Read the model definition and answer for the solid it produces. Units are mm, in the model's axes. A direction names the side the tool comes from. Round coordinates to 2 decimals unless told otherwise and drop trailing zeros. Write each loop counter-clockwise with the first axis right and the second up, starting at its lowest first coordinate (ties: lowest second). Pieces come first, ordered by that corner, then holes. Notation, with made-up numbers: (61.5, -22.75) -> (84.5, -22.75) arc R21 cw to (84.5, -9.75) -> close; hole circle Ø7 at (24.25, -25.75). An arc over 180 degrees is marked (long way). Return JSON: item names as keys, results as strings.
from build123d import *

# Parameters (mm, degrees)
F1_DEPTH = 8
F2_W     = 110
F2_H     = 20
F3_DEPTH = 25


with BuildPart() as f1:
    # F0 (on Front) → F1 (new body)
    with BuildSketch(Plane.XZ):
        Polygon((228, 40), (0, 40), (0, 20), (4, 20), (4, 0), (4, -20), (0, -20), (0, -40), (228, -40), align=None)
        Polygon((0, 20), (0, 40), (-228, 40), (-228, -40), (0, -40), (0, -20), (-95, -20), (-95, 20), align=None)
    extrude(amount=F1_DEPTH)

    # F2 (on face) → F3 (cut)
    with BuildSketch(Plane.XZ.offset(8)):
        with Locations((-173, 30)):
            Rectangle(F2_W, F2_H)
        with Locations((173, 30)):
            Rectangle(F2_W, F2_H)
    extrude(amount=-F3_DEPTH, mode=Mode.SUBTRACT)


solid = f1.part
Item 1: Straight lines are drawn through the part: L1, parallel to X at y = -2, z = 4.5; L2, parallel to Z at x = -46.5, y = -6.75; L3, parallel to X at y = -4.5, z = 22. For each, find the intervals that lie inside material, in ascending order. Write a range as [from, to].
Worked answers:
{"L1": "x = [-228, -95], [4, 228]", "L2": "z = [-40, -20], [20, 40]", "L3": "x = [-118, 118]"}
Item 2: A tool of negligible diameter and unlimited length cuts with its end or side. For faces 1 (the flat face through (2, -4, 40)), 2 (the flat face through (172, -4, 20)), 3 (the flat face through (-95, -4, 0)), 4 (the flat face through (-118, -4, 30)), from which of +Z, -Z, +X, -X, +Y, -Y can it reach the whole face along a straight path? Write none if from no direction.
Worked answers:
{"face 1": "+Z, +X, -X, +Y, -Y", "face 2": "+Z, +X, +Y, -Y", "face 3": "+Y, -Y", "face 4": "+Z, -X, +Y, -Y"}
Item 3: Flat-ended cylindrical pins translate along their axes: pin 1 (4 mm diameter, centred on x = 181, y = -6, fed in from +Z); pin 2 (4 mm diameter, centred on y = -3.5, z = 28, fed in from -X). Find the tip coordinate at first contact, or state that the pin passes through.
Worked answers:
{"pin 1": "stops at z = 20", "pin 2": "stops at x = -118"}
Item 4: For a pull along X with two mould halves and no side action, classify faces 5 (the flat face through (-228, -4, -10)), 6 (the flat face through (118, -4, 30)), 7 (the flat face through (-3, 0, -26)), 8 (the flat face through (-45, -4, -20)) as released by +X, released by -X, zero draft, split by the parting line, or undercut.
Worked answers:
{"face 5": "released by -X", "face 6": "released by +X", "face 7": "zero draft", "face 8": "undercut"}
Item 5: Section D-D (x = -189) is taken. Give the vertices of the cut face in (y, z), then the cut area to 3 significant figures.
Worked answers:
{"outline": "(-8, -40) -> (0, -40) -> (0, 20) -> (-8, 20) -> close", "area": "480 mm2"}
Item 6: Section B-B (z = 3) is taken. Give the vertices of the cut face in (x, y).
Worked answers:
{"outline": "(-228, -8) -> (-95, -8) -> (-95, 0) -> (-228, 0) -> close; (4, -8) -> (228, -8) -> (228, 0) -> (4, 0) -> close"}
Item 7: Section A-A (x = -11) is taken. Give the vertices of the cut face in (y, z).
Worked answers:
{"outline": "(-8, -40) -> (0, -40) -> (0, -20) -> (-8, -20) -> close; (-8, 20) -> (0, 20) -> (0, 40) -> (-8, 40) -> close"}
Item 8: Section C-C (y = -3.5) is taken. Give the vertices of the cut face in (x, z), then the cut area to 3 significant figures.
Worked answers:
{"outline": "(-228, -40) -> (228, -40) -> (228, 20) -> (118, 20) -> (118, 40) -> (-118, 40) -> (-118, 20) -> (-228, 20) -> close; hole (-95, -20) -> (4, -20) -> (4, 20) -> (-95, 20) -> close", "area": "28,100 mm2"}
